from build123d import *

# Parameters (mm, degrees)
SKETCH1_W                                           = 229
SKETCH1_H                                           = 120
BOSS_EXTRUDE1_DEPTH                                 = 7.5
SKETCH4_W                                           = 20.632503002
SKETCH4_H                                           = 53.730004003
BOSS_EXTRUDE2_DEPTH                                 = 15
CUT_EXTRUDE1_REACH                                  = 239.205
SKETCH5_W                                           = 61.75
SKETCH5_H                                           = 15
SKETCH5_H_2                                         = 25
CUT_EXTRUDE4_REACH                                  = 239.205
SKETCH8_R                                           = 8
LPATTERN2_COUNT                                     = 4
LPATTERN2_PITCH                                     = 65.677
LPATTERN2_COUNT_DIR2                                = 2
LPATTERN2_PITCH_DIR2                                = 88
F_9_0_9_DIAMETER_HOLE1_D                            = 9
CBORE_FOR_M8_HEX_SOCKET_HEAD_CAP_SCREW1_D           = 8.4
CBORE_FOR_M8_HEX_SOCKET_HEAD_CAP_SCREW1_CBORE_D     = 15
CBORE_FOR_M8_HEX_SOCKET_HEAD_CAP_SCREW1_CBORE_DEPTH = 8.6
F_8_0MM_DOWEL_HOLE1_D                               = 8
SKETCH18_W                                          = 120
SKETCH18_H                                          = 15
BOSS_EXTRUDE3_DEPTH                                 = 30
CUT_EXTRUDE5_REACH                                  = 268.282
SKETCH19_W                                          = 15
SKETCH19_H                                          = 36


with BuildPart() as part:
    # Sketch1 → Boss-Extrude1 (new, symmetric)
    with BuildSketch(Plane(origin=(0, 0, 0), x_dir=(1, 0, 0), z_dir=(0, 1, 0))):
        with Locations((-114.5, 0)):
            Rectangle(SKETCH1_W, SKETCH1_H)
    extrude(amount=BOSS_EXTRUDE1_DEPTH, both=True)

    # Sketch4 → Boss-Extrude2 (add)
    with BuildSketch(Plane(origin=(0, 7.5, 0), x_dir=(1, 0, 0), z_dir=(0, 1, 0))):
        with Locations((10.316251501, 33.134997999)):
            Rectangle(SKETCH4_W, SKETCH4_H)
    extrude(amount=-BOSS_EXTRUDE2_DEPTH)

    # Sketch5 → Cut-Extrude1 (cut, up to next)
    with BuildSketch(Plane(origin=(0, 7.5, 0), x_dir=(1, 0, 0), z_dir=(0, 1, 0)), mode=Mode.PRIVATE) as cut_extrude1_sk1:
        with Locations((-98.875, 9.852366083)):
            Rectangle(SKETCH5_W, SKETCH5_H)
    cut_extrude1_tool1 = extrude(cut_extrude1_sk1.sketch, amount=-CUT_EXTRUDE1_REACH, mode=Mode.PRIVATE) & part.part
    # Sketch5 → Cut-Extrude1 (cut, up to next)
    with BuildSketch(Plane(origin=(0, 7.5, 0), x_dir=(1, 0, 0), z_dir=(0, 1, 0)), mode=Mode.PRIVATE) as cut_extrude1_sk2:
        with Locations((-18.875, 20.69101)):
            Rectangle(SKETCH5_W, SKETCH5_H)
    cut_extrude1_tool2 = extrude(cut_extrude1_sk2.sketch, amount=-CUT_EXTRUDE1_REACH, mode=Mode.PRIVATE) & part.part
    # Sketch5 → Cut-Extrude1 (cut, up to next)
    with BuildSketch(Plane(origin=(0, 7.5, 0), x_dir=(1, 0, 0), z_dir=(0, 1, 0)), mode=Mode.PRIVATE) as cut_extrude1_sk3:
        with Locations((-178.875, 16.78)):
            Rectangle(SKETCH5_W, SKETCH5_H_2)
    cut_extrude1_tool3 = extrude(cut_extrude1_sk3.sketch, amount=-CUT_EXTRUDE1_REACH, mode=Mode.PRIVATE) & part.part
    add(cut_extrude1_tool1.solids().sort_by_distance((-98.875, 7.5, -9.852366))[0], mode=Mode.SUBTRACT)
    add(cut_extrude1_tool2.solids().sort_by_distance((-18.875, 7.5, -20.69101))[0], mode=Mode.SUBTRACT)
    add(cut_extrude1_tool3.solids().sort_by_distance((-178.875, 7.5, -16.78))[0], mode=Mode.SUBTRACT)

    # Sketch8 → Cut-Extrude4 (cut, up to next)
    with BuildSketch(Plane(origin=(0, 7.5, 0), x_dir=(1, 0, 0), z_dir=(0, 1, 0)), mode=Mode.PRIVATE) as cut_extrude4_sk1:
        with Locations(Location((-213, 44, 0), (0, 0, 270))):
            Circle(SKETCH8_R)
    cut_extrude4_tool1 = extrude(cut_extrude4_sk1.sketch, amount=-CUT_EXTRUDE4_REACH, mode=Mode.PRIVATE) & part.part
    cut_extrude4 = cut_extrude4_tool1.solids().sort_by_distance((-213, 7.5, -44))[0]
    add(cut_extrude4, mode=Mode.SUBTRACT)

    # LPattern2: Cut-Extrude4 4 × 2
    with Locations(*[(i * LPATTERN2_PITCH, 0, j * LPATTERN2_PITCH_DIR2) for i in range(LPATTERN2_COUNT) for j in range(LPATTERN2_COUNT_DIR2) if (i, j) != (0, 0)]):
        add(cut_extrude4, mode=Mode.SUBTRACT)

    # Ø9.0 (9) Diameter Hole1 (through all)
    with Locations(Plane(origin=(0, 7.5, 0), x_dir=(1, 0, 0), z_dir=(0, 1, 0))):
        with Locations((-179, -14.72), (-139, -14.72), (-99, -14.72), (-59, -14.72), (-19, -14.72)):
            Hole(F_9_0_9_DIAMETER_HOLE1_D / 2)

    # CBORE for M8 Hex Socket Head Cap Screw1 (through all)
    with Locations(Plane(origin=(0, -7.5, 0), x_dir=(-1, 0, 0), z_dir=(0, -1, 0))):
        with Locations((38.969, 45), (190, 45), (190, -45), (38.969, -45)):
            CounterBoreHole(CBORE_FOR_M8_HEX_SOCKET_HEAD_CAP_SCREW1_D / 2, CBORE_FOR_M8_HEX_SOCKET_HEAD_CAP_SCREW1_CBORE_D / 2, CBORE_FOR_M8_HEX_SOCKET_HEAD_CAP_SCREW1_CBORE_DEPTH)

    # Ø8.0mm Dowel Hole1 (through all)
    with Locations(Plane(origin=(0, -7.5, 0), x_dir=(-1, 0, 0), z_dir=(0, -1, 0))):
        with Locations((174.5, -45), (54.469, 45)):
            Hole(F_8_0MM_DOWEL_HOLE1_D / 2)

    # Sketch18 → Boss-Extrude3 (add)
    with BuildSketch(Plane.ZY.offset(229)):
        Rectangle(SKETCH18_W, SKETCH18_H)
    extrude(amount=BOSS_EXTRUDE3_DEPTH)

    # Sketch19 → Cut-Extrude5 (cut, up to next)
    with BuildSketch(Plane(origin=(0, 7.5, 0), x_dir=(1, 0, 0), z_dir=(0, 1, 0)), mode=Mode.PRIVATE) as cut_extrude5_sk1:
        with Locations((-236.6, -7.72)):
            Rectangle(SKETCH19_W, SKETCH19_H)
    cut_extrude5_tool1 = extrude(cut_extrude5_sk1.sketch, amount=-CUT_EXTRUDE5_REACH, mode=Mode.PRIVATE) & part.part
    add(cut_extrude5_tool1.solids().sort_by_distance((-236.6, 7.5, 7.72))[0], mode=Mode.SUBTRACT)


solid = part.part
Work out the finished part from the listing and answer in its coordinate system (mm). A direction names the side the tool comes from. Coordinates: 2 decimals unless noted, no trailing zeros. Loops run counter-clockwise (first coordinate to the right, second up) from the corner with the lowest first, then second, coordinate; pieces in that order, holes last. Notation, with made-up numbers: (-19, 44.5) -> (-9, 44.5) arc R30 cw to (-9, 71.5) -> close; hole circle Ø11 at (-32, 14). An arc over 180 degrees is marked (long way). Answer as CSV lines item,"result".
1) The part is cut by section A-A (x = -213). Give the vertices of the cut face in (y, z), and give its area (3 significant figures).
A:
outline,"(-7.5, -60) -> (7.5, -60) -> (7.5, -52) -> (-7.5, -52) -> close; (-7.5, -36) -> (7.5, -36) -> (7.5, 36) -> (-7.5, 36) -> close; (-7.5, 52) -> (7.5, 52) -> (7.5, 60) -> (-7.5, 60) -> close"
area,"1,320 mm²"
2) Flat-ended cylindrical pins translate along their axes: pin 1 (7.5 mm diameter, centred on x = -190, z = -45, fed in from +Y); pin 2 (8 mm diameter, centred on y = 0, z = 19.5, fed in from +X); pin 3 (7.5 mm diameter, centred on x = -190, z = 41.5, fed in from -Y). Find the tip coordinate at first contact, or state that the pin passes through.
A:
pin 1,"passes through"
pin 2,"stops at x = 0"
pin 3,"stops at y = 1.1"
3) The part is cut by section C-C (x = -110.5). Give the vertices of the cut face in (y, z), and give its area (4 significant figures).
A:
outline,"(-7.5, -60) -> (7.5, -60) -> (7.5, -17.35) -> (-7.5, -17.35) -> close; (-7.5, -2.35) -> (7.5, -2.35) -> (7.5, 60) -> (-7.5, 60) -> close"
area,"1,575 mm²"
4) Straight lines are drawn through the part: probe 1 along X at (y, z) = (-6.5, -9); probe 2 along X at (y, z) = (-6.5, -19); probe 3 along Z at (x, y) = (-190, -4.5). For each, find the intervals that lie inside material, in ascending order.
A:
probe 1,"x = -259 to -244.1, -229.1 to -209.75, -148 to -129.75, -68 to 20.63"
probe 2,"x = -259 to -209.75, -148 to -49.75, 12 to 20.63"
probe 3,"z = -60 to -52.5, -37.5 to -29.28, -4.28 to 37.5, 52.5 to 60"
5) For faces 1 (the face through (-37.34, -3.26, -37.68)), 2 (the face through (20.633, 0, -33)), 3 (the face through (-99, 0, -17.352)), determine the directions among +Z, -Z, +X, -X, +Y, -Y from which every point of the face is accessible in a straight line to the end or side of a thin tool.
A:
face 1,"-Y"
face 2,"+Z, -Z, +X, +Y, -Y"
face 3,"+Y, -Y"
6) For a pull along Z with two mould halves and no side action, classify faces 4 (the face through (0, 0, 27)), 5 (the face through (10, 0, -6.27)), 6 (the face through (-19, 0, -13.191)) as released by +Z, released by -Z, zero draft, split by the parting line, or undercut.
A:
face 4,"zero draft"
face 5,"released by +Z"
face 6,"undercut"
7) The part is cut by section B-B (z = 2). Give the vertices of the cut face in (x, y), and give its area (3 significant figures).
A:
outline,"(-259, -7.5) -> (-244.1, -7.5) -> (-244.1, 7.5) -> (-259, 7.5) -> close; (-229.1, -7.5) -> (0, -7.5) -> (0, 7.5) -> (-229.1, 7.5) -> close"
area,"3,660 mm²"
